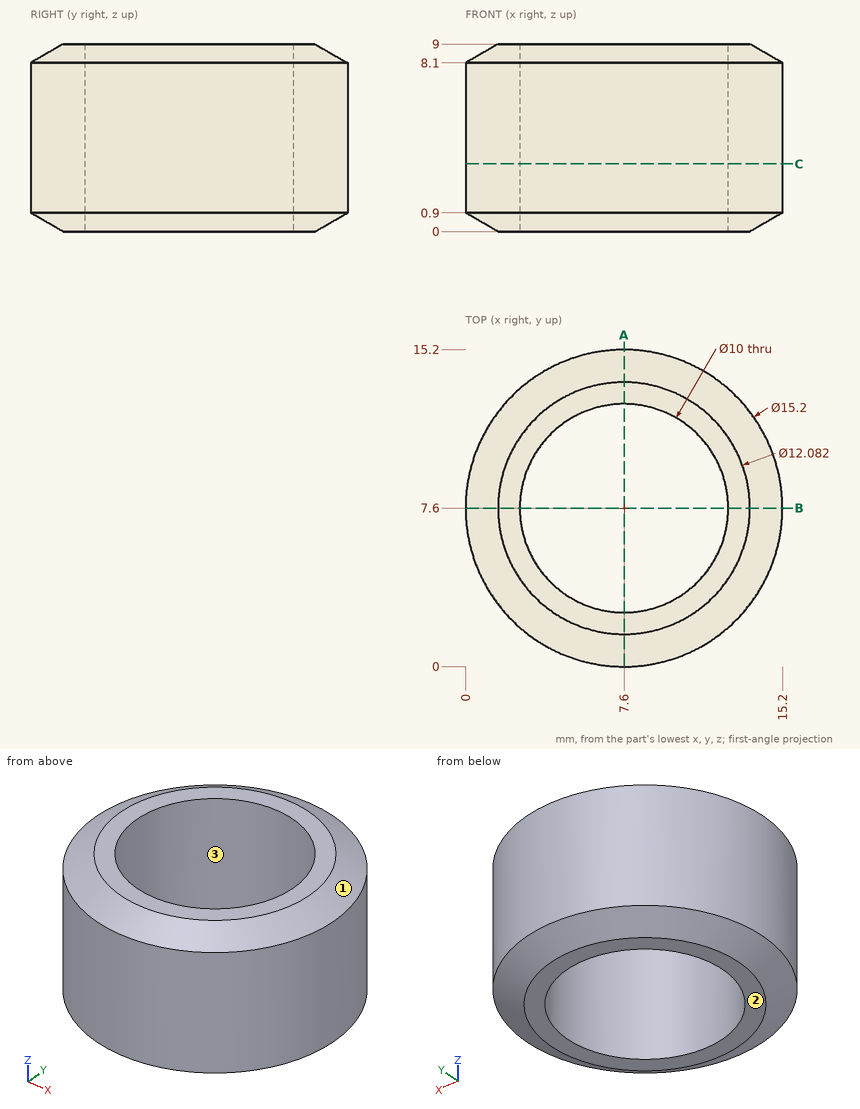
The figure shows three views and two pictorial views of one solid part (mm, origin at its lowest corner). Answer the questions. Give positions to 0.01 mm unless a question says otherwise; leave off trailing zeros. Write each loop counter-clockwise with the first axis right and the second up, starting at its lowest first coordinate (ties: lowest second). Pieces come first, ordered by that corner, then holes. Notation, with made-up numbers: (73, 42.5) -> (100, 42.5) arc R16 cw to (100, 70.5) -> close; hole circle Ø2 at (4, 84.5). An arc over 180 degrees is marked (long way). Write each question's results on one line, items separated by ' | '.
1. Determine the mould class of the marked faces 1, 2 and 3 for opening direction Y: +Y half, -Y half, draft (parallel to the pull), parting line (faces both ways), or undercut.
Data:
face 1: parting line | face 2: draft | face 3: undercut
2. Each of these flat-tipped pins is pushed along its axis until it touches: pin 1 Ø2 at (y, z) = (3, 3.5) entering from +X; pin 2 Ø3 at (y, z) = (3.5, 2) entering from -X; pin 3 Ø3 at (x, z) = (10.5, 3) entering from -Y. Where does it stop, or does it pass through?
Data:
pin 1: x = 14.29 | pin 2: x = 0.46 | pin 3: y = 0.13
3. Straight lines are drawn through the part: L1, parallel to Y at x = 7.6, z = 3; L2, parallel to X at y = 3, z = 1.75; L3, parallel to X at y = 12, z = 4 (1 decimal). For each, find the intervals that lie inside material, in ascending order.
Data:
L1: 0 to 2.6, 12.6 to 15.2 | L2: 1.55 to 5.64, 9.56 to 13.65 | L3: 1.4 to 5.2, 10 to 13.8
4. Find section C-C on z = 3.25. Determine the outline of the cut face in (x, y).
Data:
outline: circle Ø15.2 at (7.6, 7.6); hole circle Ø10 at (7.6, 7.6)
5. Find section A-A on x = 7.6. Determine the outline of the cut face in (y, z).
Data:
outline: (0, 0.9) -> (1.56, 0) -> (2.6, 0) -> (2.6, 9) -> (1.56, 9) -> (0, 8.1) -> close; (12.6, 0) -> (13.64, 0) -> (15.2, 0.9) -> (15.2, 8.1) -> (13.64, 9) -> (12.6, 9) -> close
